```python
from build123d import *

# Parameters (mm, degrees)
SKETCH_1_W          = 20
SKETCH_1_H          = 10
EXTRUDE_1_DEPTH     = 5
SKETCH_2_R          = 1.5
CUT_EXTRUDE_1_DEPTH = 16
SKETCH_3_W          = 3
SKETCH_3_H          = 10
EXTRUDE_2_DEPTH     = 8
SKETCH_6_W          = 20
SKETCH_6_H          = 10
EXTRUDE_4_DEPTH     = 3
SKETCH_7_R          = 1.5
CUT_EXTRUDE_3_DEPTH = 24.157072354
FILLET_2_R          = 3
FILLET_4_R          = 2
SKETCH_11_W         = 10
SKETCH_11_H         = 11
EXTRUDE_7_DEPTH     = 1
FILLET_8_R          = 3
SKETCH_12_W         = 20
SKETCH_12_H         = 10
EXTRUDE_8_DEPTH     = 1


with BuildPart() as part:
    # 草图1 → 凸台-拉伸1 (new body)
    with BuildSketch(Plane(origin=(0, 0, 0), x_dir=(1, 0, 0), z_dir=(0, 1, 0))):
        Rectangle(SKETCH_1_W, SKETCH_1_H)
    extrude(amount=EXTRUDE_1_DEPTH)

    # 草图2 → 切除-拉伸1 (cut, through all)
    with BuildSketch(Plane.XY.offset(5)):
        with Locations((-6, 2.5)):
            Circle(SKETCH_2_R)
        with Locations((6, 2.5)):
            Circle(SKETCH_2_R)
    extrude(amount=-CUT_EXTRUDE_1_DEPTH, mode=Mode.SUBTRACT)

    # 草图3 → 凸台-拉伸2 (add)
    with BuildSketch(Plane.XZ):
        Rectangle(SKETCH_3_W, SKETCH_3_H)
    extrude(amount=EXTRUDE_2_DEPTH)

    # 草图6 → 凸台-拉伸4 (add)
    with BuildSketch(Plane.XZ.offset(8)):
        with Locations((-8.5, 0)):
            Rectangle(SKETCH_6_W, SKETCH_6_H)
    extrude(amount=EXTRUDE_4_DEPTH)

    # 草图7 → 切除-拉伸3 (cut, through all)
    with BuildSketch(Plane(origin=(0, -8, 0), x_dir=(1, 0, 0), z_dir=(0, 1, 0))):
        with Locations(Location((-14.5, 0, 0), (0, 0, 270))):
            Circle(SKETCH_7_R)
        with Locations(Location((-6.5, 0, 0), (0, 0, 270))):
            Circle(SKETCH_7_R)
    extrude(amount=-CUT_EXTRUDE_3_DEPTH, mode=Mode.SUBTRACT)

    # 圆角2
    fillet_2_edges = [part.edges().sort_by_distance(p)[0] for p in [
        (-1.5, 0, 0),
    ]]
    fillet(fillet_2_edges, radius=FILLET_2_R)

    # 圆角4
    fillet_4_edges = [part.edges().sort_by_distance(p)[0] for p in [
        (-1.5, -8, 0),
    ]]
    fillet(fillet_4_edges, radius=FILLET_4_R)

    # 草图11 → 凸台-拉伸7 (add)
    with BuildSketch(Plane(origin=(1.5, 0, 0), x_dir=(0, 0, -1), z_dir=(1, 0, 0))):
        with Locations((0, -5.5)):
            Rectangle(SKETCH_11_W, SKETCH_11_H)
    extrude(amount=EXTRUDE_7_DEPTH)

    # 圆角8
    fillet_8_edges = [part.edges().sort_by_distance(p)[0] for p in [
        (2.5, 0, 0),
    ]]
    fillet(fillet_8_edges, radius=FILLET_8_R)

    # 草图12 → 凸台-拉伸8 (add)
    with BuildSketch(Plane(origin=(0, 5, 0), x_dir=(1, 0, 0), z_dir=(0, 1, 0))):
        Rectangle(SKETCH_12_W, SKETCH_12_H)
    extrude(amount=EXTRUDE_8_DEPTH)


solid = part.part
```
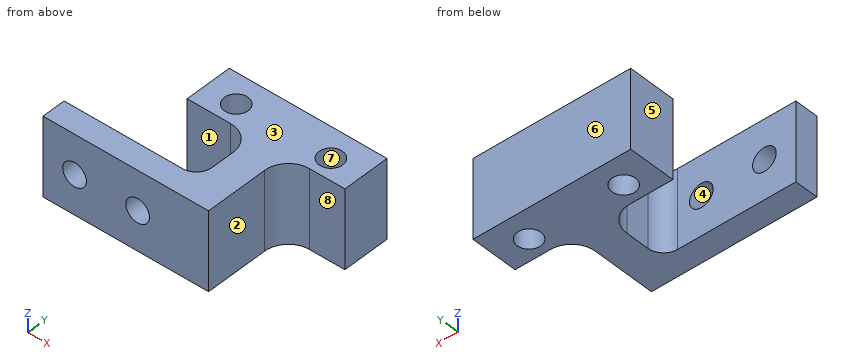
CAD build for the part. Positions are in the model's coordinates, mm. Face numbers are marked on the shaded views. A direction names the side the tool comes from. Give positions to 0.01 mm unless a question says otherwise; leave off trailing zeros. Loops run counter-clockwise (first coordinate to the right, second up) from the corner with the lowest first, then second, coordinate; pieces in that order, holes last. Notation, with made-up numbers: M 39,37.5 L 55,37.5 A23 ccw 55,69.5 Z; hole C -14,82.5 d11. An arc over 180 degrees is marked long. Use one line per item in the form item = value.
Item 1: Two-plate mould, pull along Y, no slides. Class the marked faces 5, 6, 7 and 8: pulls with the +Y half, pulls with the -Y half, needs draft (parallel to the pull), parting line crosses it, or undercut.
Determined:
face_5 = needs draft
face_6 = pulls with the +Y half
face_7 = undercut
face_8 = pulls with the -Y half
Item 2: Slice it at C-C (y = 2.5). List the corners of the cut face in (x, z), plus the area to 3 significant figures.
Determined:
outline = M -10,-5 L -7.5,-5 L -7.5,5 L -10,5 Z; M -4.5,-5 L 4.5,-5 L 4.5,5 L -4.5,5 Z; M 7.5,-5 L 10,-5 L 10,5 L 7.5,5 Z
area = 140 mm2
Item 3: Which spindle directions (+Z, -Z, +X, -X, +Y, -Y) get a long thin tool onto all of the face, cutting with end or side? Do the marked faces 1, 2, 3 and 4. Say none if no direction does.
Determined:
face_1 = +Z, -Z, -X
face_2 = +Z, -Z, +X, -Y
face_3 = +Z, +X, -X, +Y, -Y
face_4 = -Y
Item 4: Slice it at B-B (x = -14.5). List the corners of the cut face in (y, z).
Determined:
outline = M -11,-5 L -8,-5 L -8,-1.5 L -11,-1.5 Z; M -11,1.5 L -8,1.5 L -8,5 L -11,5 Z
Item 5: Flat gauge pins, fed straight in: pin 1 (4 mm diameter, centred on y = -6.5, z = -1.5, fed in from +X); pin 2 (1.8 mm diameter, centred on y = 4, z = 0.5, fed in from -X); pin 3 (3.5 mm diameter, centred on x = -14.5, z = 0, fed in from -Y); pin 4 (2 mm diameter, centred on x = 8, z = 0.5, fed in from -Y). Where does each tip first touch, or does it go through?
Determined:
pin_1 = 2.5
pin_2 = -10
pin_3 = -11
pin_4 = 0
Item 6: Drill centre lines: probe 1 along Y at (x, z) = (-6, -1.5); probe 2 along X at (y, z) = (-9.05, 0); probe 3 along X at (y, z) = (1.75, -1.5). Where is each one in solid material? Low to high. Write a range as from..to.
Determined:
probe_1 = -11..-8, 0..1, 4..6
probe_2 = -18.5..-16, -13..-8, -5..2.5
probe_3 = -10..-7.3, -4.7..4.7, 7.3..10
Item 7: Slice it at D-D (x = -6). List the corners of the cut face in (y, z).
Determined:
outline = M -11,-5 L -8,-5 L -8,-1.41 L -11,-1.41 Z; M -11,1.41 L -8,1.41 L -8,5 L -11,5 Z; M 0,-5 L 1,-5 L 1,5 L 0,5 Z; M 4,-5 L 6,-5 L 6,5 L 4,5 Z
Item 8: Slice it at A-A (z = 0). List the corners of the cut face in (x, y).
Determined:
outline = M -18.5,-11 L -16,-11 L -16,-8 L -18.5,-8 Z; M -13,-11 L -8,-11 L -8,-8 L -13,-8 Z; M -10,0 L -4.5,0 A3 cw -1.5,-3 L -1.5,-6 A2 cw -3.5,-8 L -5,-8 L -5,-11 L 2.5,-11 L 2.5,-3 A3 cw 5.5,0 L 10,0 L 10,6 L -10,6 Z; hole C -6,2.5 d3; hole C 6,2.5 d3
